The listing builds one solid part. Answer for the finished solid, in the listing's coordinates (mm). A direction names the side the tool comes from. Round coordinates to 2 decimals unless told otherwise and drop trailing zeros. Order: outer loops, then holes, each group sorted by start corner. A loop starts at its lowest first (then second) coordinate and runs counter-clockwise, first axis right, second up. Notation, with made-up numbers: (-38.5, 4.5) - (-17.5, 4.5) arc R23 ccw to (-17.5, 14.5) - close; hole circle Ø4 at (-17, -7.5). An arc over 180 degrees is marked (long way). Use CSV: the item, a comma, the result in double quotes. Start each with the question number.
Item 1: Determine the mould class of faces 4 (the flat face through (-75.605, 25, 31)), 5 (the flat face through (-80.605, 23, 26)), 6 (the flat face through (-78, 45, 31)) for opening direction X: +X half, -X half, draft (parallel to the pull), parting line (faces both ways), or undercut.
Item 2: Find section C-C, the plane y = 21.5. Give the vertices of the cut face in (x, z), plus the area to 3 significant figures.
Item 3: Find section A-A, the plane y = 38. Give the vertices of the cut face in (x, z).
Item 4: Flat-ended cylindrical pins translate along their axes: P1, Ø1.5, axis at x = 95.5, y = 41, coming from the -Z side; P2, Ø5, axis at x = -47, z = 35, coming from the +Y side; P3, Ø4, axis at x = -24, z = -42, coming from the +Y side. Find the tip coordinate at first contact, or state that the pin passes through.
Item 5: Straight lines are drawn through the part: line 1 along X through (y, z) = (7.5, -15); line 2 along Z through (x, y) = (53, 16); line 3 along Y through (x, z) = (-22, 19). For each, find the intervals that lie inside material, in ascending order. Write a range as [from, to].
Item 6: Find section B-B, the plane z = 48. Give the vertices of the cut face in (x, y), plus the area to 3 significant figures.
Item 7: For faces 1 (the flat face through (9, 3, 99.758)), 2 (the flat face through (11, 20, -40.242)), 3 (the flat face through (-78, 40, -40.242)), determine the directions among +Z, -Z, +X, -X, +Y, -Y from which every point of the face is accessible in a straight line to the end or side of a thin tool.
```python
from build123d import *

# Parameters (mm, degrees)
SKETCH1_W           = 180
SKETCH1_H           = 150
BOSS_EXTRUDE1_DEPTH = 5
SKETCH5_W           = 5
SKETCH5_H           = 40
BOSS_EXTRUDE2_DEPTH = 140
SKETCH13_W          = 5
SKETCH13_H          = 30
BOSS_EXTRUDE9_DEPTH = 180


with BuildPart() as part:
    # Sketch1 → Boss-Extrude1 (new body)
    with BuildSketch(Plane(origin=(0, 0, 0), x_dir=(1, 0, 0), z_dir=(0, 1, 0))):
        with Locations((9.394856278, -24.757942511)):
            Rectangle(SKETCH1_W, SKETCH1_H)
    extrude(amount=BOSS_EXTRUDE1_DEPTH)

    # Sketch5 → Boss-Extrude2 (add)
    with BuildSketch(Plane.XY.offset(99.757942511)):
        with Locations((-78.105143722, 25)):
            Rectangle(SKETCH5_W, SKETCH5_H)
        with Locations((96.894856278, 25)):
            Rectangle(SKETCH5_W, SKETCH5_H)
    extrude(amount=-BOSS_EXTRUDE2_DEPTH)

    # Sketch13 → Boss-Extrude9 (add)
    with BuildSketch(Plane(origin=(99.394856278, 0, 0), x_dir=(0, 0, -1), z_dir=(1, 0, 0))):
        with Locations((42.742057489, 20)):
            Rectangle(SKETCH13_W, SKETCH13_H)
    extrude(amount=-BOSS_EXTRUDE9_DEPTH)


solid = part.part
```
Worked out:
1,face 4,"undercut"
1,face 5,"-X half"
1,face 6,"draft"
2,outline,"(-80.61, -45.24) - (99.39, -45.24) - (99.39, 99.76) - (94.39, 99.76) - (94.39, -40.24) - (-75.61, -40.24) - (-75.61, 99.76) - (-80.61, 99.76) - close"
2,area,"2,300 mm²"
3,outline,"(-80.61, -40.24) - (-75.61, -40.24) - (-75.61, 99.76) - (-80.61, 99.76) - close; (94.39, -40.24) - (99.39, -40.24) - (99.39, 99.76) - (94.39, 99.76) - close"
4,P1,"stops at z = -40.24"
4,P2,"stops at y = 5"
4,P3,"stops at y = 35"
5,line 1,"x = [-80.61, -75.61], [94.39, 99.39]"
5,line 2,"z = [-45.24, -40.24]"
5,line 3,"y = [0, 5]"
6,outline,"(-80.61, 0) - (99.39, 0) - (99.39, 45) - (94.39, 45) - (94.39, 5) - (-75.61, 5) - (-75.61, 45) - (-80.61, 45) - close"
6,area,"1,300 mm²"
7,face 1,"+Z, +X, -X, +Y, -Y"
7,face 2,"+Z, +Y"
7,face 3,"-Z, +X, -X, +Y"
